Geometry check sheet. Reference: the model listing, model coordinates, mm. Round coordinates to 2 decimals unless told otherwise and drop trailing zeros. Order: outer loops, then holes, each group sorted by start corner. A loop starts at its lowest first (then second) coordinate and runs counter-clockwise, first axis right, second up.
```python
from build123d import *

# Parameters (mm, degrees)
SKETCH1_R           = 2.6
SKETCH1_R_2         = 0.5
BOSS_EXTRUDE1_DEPTH = 1.6


with BuildPart() as part:
    # Sketch1 → Boss-Extrude1 (new body)
    with BuildSketch(Plane(origin=(0, 0, 0), x_dir=(1, 0, 0), z_dir=(0, 1, 0))):
        with BuildLine():
            Line((70, -100), (-70, -100))
            ThreePointArc((-70, -100), (-91.213203436, -91.213203436), (-100, -70))
            Line((-100, -70), (-100, 70))
            ThreePointArc((-100, 70), (-91.213203436, 91.213203436), (-70, 100))
            Line((-70, 100), (70, 100))
            ThreePointArc((70, 100), (91.213203436, 91.213203436), (100, 70))
            Line((100, 70), (100, -70))
            ThreePointArc((100, -70), (91.213203436, -91.213203436), (70, -100))
        make_face()
        with Locations(Location((-82.6, 82.6, 0), (0, 0, 270))):
            Circle(SKETCH1_R, mode=Mode.SUBTRACT)
        with Locations(Location((82.6, 82.6, 0), (0, 0, 270))):
            Circle(SKETCH1_R, mode=Mode.SUBTRACT)
        with Locations(Location((82.6, -82.6, 0), (0, 0, 270))):
            Circle(SKETCH1_R, mode=Mode.SUBTRACT)
        with Locations(Location((-82.6, -82.6, 0), (0, 0, 270))):
            Circle(SKETCH1_R, mode=Mode.SUBTRACT)
        with Locations(Location((-60, 60, 0), (0, 0, 270))):
            Circle(SKETCH1_R_2, mode=Mode.SUBTRACT)
        with Locations(Location((-20, 60, 0), (0, 0, 270))):
            Circle(SKETCH1_R_2, mode=Mode.SUBTRACT)
        with Locations(Location((-20, 20, 0), (0, 0, 270))):
            Circle(SKETCH1_R_2, mode=Mode.SUBTRACT)
        with Locations(Location((-60, 20, 0), (0, 0, 270))):
            Circle(SKETCH1_R_2, mode=Mode.SUBTRACT)
        with Locations(Location((60, 20, 0), (0, 0, 270))):
            Circle(SKETCH1_R_2, mode=Mode.SUBTRACT)
        with Locations(Location((20, 20, 0), (0, 0, 270))):
            Circle(SKETCH1_R_2, mode=Mode.SUBTRACT)
        with Locations(Location((20, 60, 0), (0, 0, 270))):
            Circle(SKETCH1_R_2, mode=Mode.SUBTRACT)
        with Locations(Location((60, 60, 0), (0, 0, 270))):
            Circle(SKETCH1_R_2, mode=Mode.SUBTRACT)
        with Locations(Location((20, -20, 0), (0, 0, 270))):
            Circle(SKETCH1_R_2, mode=Mode.SUBTRACT)
        with Locations(Location((60, -20, 0), (0, 0, 270))):
            Circle(SKETCH1_R_2, mode=Mode.SUBTRACT)
        with Locations(Location((60, -60, 0), (0, 0, 270))):
            Circle(SKETCH1_R_2, mode=Mode.SUBTRACT)
        with Locations(Location((20, -60, 0), (0, 0, 270))):
            Circle(SKETCH1_R_2, mode=Mode.SUBTRACT)
        with Locations(Location((-20, -20, 0), (0, 0, 270))):
            Circle(SKETCH1_R_2, mode=Mode.SUBTRACT)
        with Locations(Location((-60, -20, 0), (0, 0, 270))):
            Circle(SKETCH1_R_2, mode=Mode.SUBTRACT)
        with Locations(Location((-20, -60, 0), (0, 0, 270))):
            Circle(SKETCH1_R_2, mode=Mode.SUBTRACT)
        with Locations(Location((-60, -60, 0), (0, 0, 270))):
            Circle(SKETCH1_R_2, mode=Mode.SUBTRACT)
    extrude(amount=BOSS_EXTRUDE1_DEPTH)


solid = part.part
```
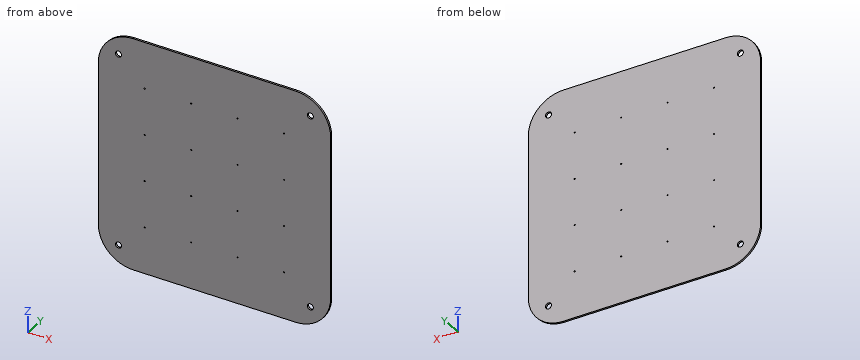
(1) Sectioned sample at B-B, the plane z = -82.6. Record the cut outline in (x, y), and give its area (3 significant figures).
Returned:
outline: (-97.23, 0) - (-85.2, 0) - (-85.2, 1.6) - (-97.23, 1.6) - close; (-80, 0) - (80, 0) - (80, 1.6) - (-80, 1.6) - close; (85.2, 0) - (97.23, 0) - (97.23, 1.6) - (85.2, 1.6) - close
area: 294 mm2
(2) Material ranges on line 1 (X direction, y = 0.8, z = 20); line 2 (X direction, y = 0.7, z = 82.6), recorded low to high.
Returned:
line 1: x = -100 to -60.5, -59.5 to -20.5, -19.5 to 19.5, 20.5 to 59.5, 60.5 to 100
line 2: x = -97.23 to -85.2, -80 to 80, 85.2 to 97.23
(3) Sectioned sample at C-C, the plane x = -87.5. Record the cut outline in (y, z), and give its area (3 significant figures).
Returned:
outline: (0, -94.37) - (1.6, -94.37) - (1.6, 94.37) - (0, 94.37) - close
area: 302 mm2
(4) Sectioned sample at A-A, the plane y = 0.55. Give the number of separate pieces and of enclosed holes in the cut face, and give its area (3 significant figures).
Returned:
separate pieces: 1
enclosed holes: 20
area: 39,100 mm2
(5) Depth check by flat-ended pin: P1, Ø4.5, axis at x = -82.6, z = -82.6, coming from the -Y side. Enter the tip coordinate at first touch or a pass-through.
Returned:
P1: passes through
